Autodesk Inventor part; units mm, degrees
ref_plane "YZ Plane" through (0, 0, 0) normal (1, 0, 0) x (0, 1, 0)
ref_plane "XZ Plane" through (0, 0, 0) normal (0, 1, 0) x (-1, 0, 0)
ref_plane "XY Plane" through (0, 0, 0) normal (0, 0, 1) x (1, 0, 0)
sketch "Sketch1" plane through (0, 0, 0) normal (0, 1, 0) x (-1, 0, 0)
  line L0 (0, -5.6886) -> (6.7556, -12.4442)
  line L1 (6.7556, -12.4442) -> (5.3414, -13.8584)
  line L2 (9.5, -18.017) -> (5.3414, -13.8584)
  line L3 (10, -18.017) -> (9.5, -18.017)
  line L4 (10, -18.017) -> (10, 0)
  line L5 (0, 0) -> (10, 0)
  line L6 (0, 0) -> (0, -5.6886)
  circle A0 centre (5, -2.8443) radius 1.339
extrude "Extrusion1" add sketch "Sketch1" along normal blind 10
sketch "Sketch2" plane through (0, 10, 0) normal (0, 1, 0) x (1, 0, 0)
  line L0 (0, 5.6886) -> (-10, 5.6886)
  line L1 (-10, 5.6886) -> (-10, 0)
  line L2 (-10, 0) -> (0, 0)
  line L3 (0, 0) -> (0, 5.6886)
extrude "Extrusion2" add sketch "Sketch2" along normal blind 20
sketch "Sketch3" plane through (0, 0, 0) normal (0, -1, 0) x (1, 0, 0)
  circle A0 centre (-5, -2.8443) radius 1.339
hole "Hole1" at (-5, 0, -2.8443) direction (0, 1, 0) diameter 4.318 depth 31 tip angle 118
sketch "Sketch4" plane through (-9.5, 0, -18.017) normal (0.7071, 0, -0.7071) x (-0.7071, 0, -0.7071)
  circle A0 centre (-2.9406, 5) radius 2.55
  point P0 (-19.4575, 0)
  dimension "d11" = 5.1
extrude "Extrusion3" cut sketch "Sketch4" against normal blind 0.1
sketch "Sketch6" plane through (-9.5, 0, -18.017) normal (0.7071, 0, -0.7071) x (-0.7071, 0, -0.7071)
  circle A0 centre (-2.9406, 5) radius 2.55
  line L0 (-5.8811, 0) -> (0, 0)
  line L1 (0, 0) -> (0, 10)
  line L2 (-5.8811, 10) -> (0, 10)
  line L3 (-5.8811, 0) -> (-5.8811, 10)
  point P0 (-19.4575, 0)
sketch "Sketch8" plane through (0, 30, 0) normal (0, 1, 0) x (1, 0, 0)
  circle A0 centre (-5, 2.8443) radius 2.159
  line L0 (0, 5.6886) -> (-10, 5.6886)
  line L1 (-10, 5.6886) -> (-10, 0)
  line L2 (-10, 0) -> (0, 0)
  line L3 (0, 0) -> (0, 5.6886)
extrude "Extrusion5" cut sketch "Sketch8" against normal blind 2
extrude "Extrusion6" add sketch "Sketch6" along normal blind 2
sketch "Sketch9" plane through (-8.0858, 0, -19.4312) normal (0.7071, 0, -0.7071) x (-0.7071, 0, -0.7071)
  line L0 (-4.9902, 1.1733) -> (-0.8909, 1.1733)
  line L1 (-0.8909, 1.1733) -> (-0.8909, 8.8267)
  line L2 (-0.8909, 8.8267) -> (-4.9902, 8.8267)
  line L3 (-4.9902, 8.8267) -> (-4.9902, 1.1733)
  line L4 (-4.9902, 1.1733) -> (-0.8909, 8.8267) construction
  line L5 (-0.8909, 1.1733) -> (-4.9902, 8.8267) construction
  point P0 (-19.4575, 0)
  point P1 (-2.9406, 5)
extrude "Extrusion7" cut sketch "Sketch9" against normal blind 0.2
sketch "Sketch10" plane through (-8.2272, 0, -19.2898) normal (0.7071, 0, -0.7071) x (-0.7071, 0, -0.7071)
  line L0 (-4.9902, 8.3098) -> (-0.8909, 8.3098)
  line L1 (-0.8909, 8.3098) -> (-0.8909, 8.8267)
  line L2 (-0.8909, 8.8267) -> (-4.9902, 8.8267)
  line L3 (-4.9902, 8.8267) -> (-4.9902, 8.3098)
  point P0 (-19.4575, 0)
extrude "Extrusion8" cut sketch "Sketch10" against normal blind 0.3
sketch "Sketch11" plane through (-8.2272, 0, -19.2898) normal (0.7071, 0, -0.7071) x (-0.7071, 0, -0.7071)
  line L0 (-4.9902, 1.1733) -> (-0.8909, 1.1733)
  line L1 (-0.8909, 1.1733) -> (-0.8909, 1.613)
  line L2 (-0.8909, 1.613) -> (-4.9902, 1.613)
  line L3 (-4.9902, 1.613) -> (-4.9902, 1.1733)
  point P0 (-19.4575, 0)
extrude "Extrusion9" cut sketch "Sketch11" against normal blind 0.3
properties part number "sampleHolder_v3"
Part model, mm, in its own coordinate system. A direction names the side the tool comes from. Give positions to 0.01 mm unless a question says otherwise; leave off trailing zeros. Order: outer loops, then holes, each group sorted by start corner. A loop starts at its lowest first (then second) coordinate and runs counter-clockwise, first axis right, second up. Notation, with made-up numbers: (-16.5, -25.75) - (-3.5, -25.75) arc R21 ccw to (-3.5, -18.75) - close; hole circle Ø8 at (-36.5, 58). An arc over 180 degrees is marked (long way). Use a Markdown table: item, result.
1) Saw through at C-C on x = -1.25. List the corners of the cut face in (y, z).
Checked values:
| item | result |
|---|---|
| outline | (0, -6.94) - (10, -6.94) - (10, -5.69) - (28, -5.69) - (28, 0) - (0, 0) - close |
2) Probe L1, parallel to Y at x = -6.25, z = -17.25; L2, parallel to Z at x = -5, y = 18.75; L3, parallel to Z at x = -5, y = 5.75. List the from-to ranges inside material, lowest first. Write a range as from..to.
Checked values:
| item | result |
|---|---|
| L1 | 0..1.17, 1.61..2.45, 7.55..8.31, 8.83..10 |
| L2 | -5.69..-5, -0.69..0 |
| L3 | -14.91..-14.2, -10.69..-5, -0.69..0 |
3) Saw through at D-D on z = -6.25. List the corners of the cut face in (x, y).
Checked values:
| item | result |
|---|---|
| outline | (-10, 0) - (-0.56, 0) - (-0.56, 10) - (-10, 10) - close |
4) 3-axis set-ups, long thin cutter, end or side, ignore diameter. For faces 1 (the flat face through (-7, 10, -10)), 2 (the flat face through (-6.1, 4.9, -13.1)), 3 (the flat face through (-7.47, 5.04, -15.84)), 4 (the flat face through (-10, 11, -5)), 5 (the flat face through (-7.826, 6.181, -19.171)): which of +Z, -Z, +X, -X, +Y, -Y reach the whole face in a straight line?
Checked values:
| item | result |
|---|---|
| face 1 | -Z, +X, -X, +Y |
| face 2 | +X, +Y, -Y |
| face 3 | none |
| face 4 | +Z, -Z, -X, +Y, -Y |
| face 5 | -Z, +X, +Y, -Y |
5) Saw through at A-A on z = -3.5. List the corners of the cut face in (x, y), plus the area to 3 significant figures.
Checked values:
| item | result |
|---|---|
| outline | (-10, 0) - (-7.06, 0) - (-7.06, 28) - (-10, 28) - close; (-2.94, 0) - (0, 0) - (0, 28) - (-2.94, 28) - close |
| area | 165 mm² |
6) Two-plate mould, pull along Z, no slides. Class faces 6 (the flat face through (-8.803, 4.93, -18.714)), 7 (the flat face through (-5, 0, -8)), 8 (the flat face through (-4.6, 4.9, -14.6)): +Z half, -Z half, draft (parallel to the pull), parting line (faces both ways), or undercut.
Checked values:
| item | result |
|---|---|
| face 6 | -Z half |
| face 7 | draft |
| face 8 | undercut |
7) Flat gauge pins, fed straight in: P1, Ø2, axis at x = -2, y = 14.5, coming from the -Z side; P2, Ø1, axis at x = -5.5, z = -18, coming from the +Y side; P3, Ø1, axis at x = -7, z = -7, coming from the +Y side; P4, Ø5, axis at y = 7.5, z = -11, coming from the +X side. Where does each tip first touch, or does it go through?
Checked values:
| item | result |
|---|---|
| P1 | z = -5.69 |
| P2 | through |
| P3 | y = 10 |
| P4 | x = -2.81 |
8) Saw through at B-B on y = 14.5. List the corners of the cut face in (x, z), plus the area to 3 significant figures.
Checked values:
| item | result |
|---|---|
| outline | (-10, -5.69) - (0, -5.69) - (0, 0) - (-10, 0) - close; hole circle Ø4.32 at (-5, -2.84) |
| area | 42.2 mm² |
